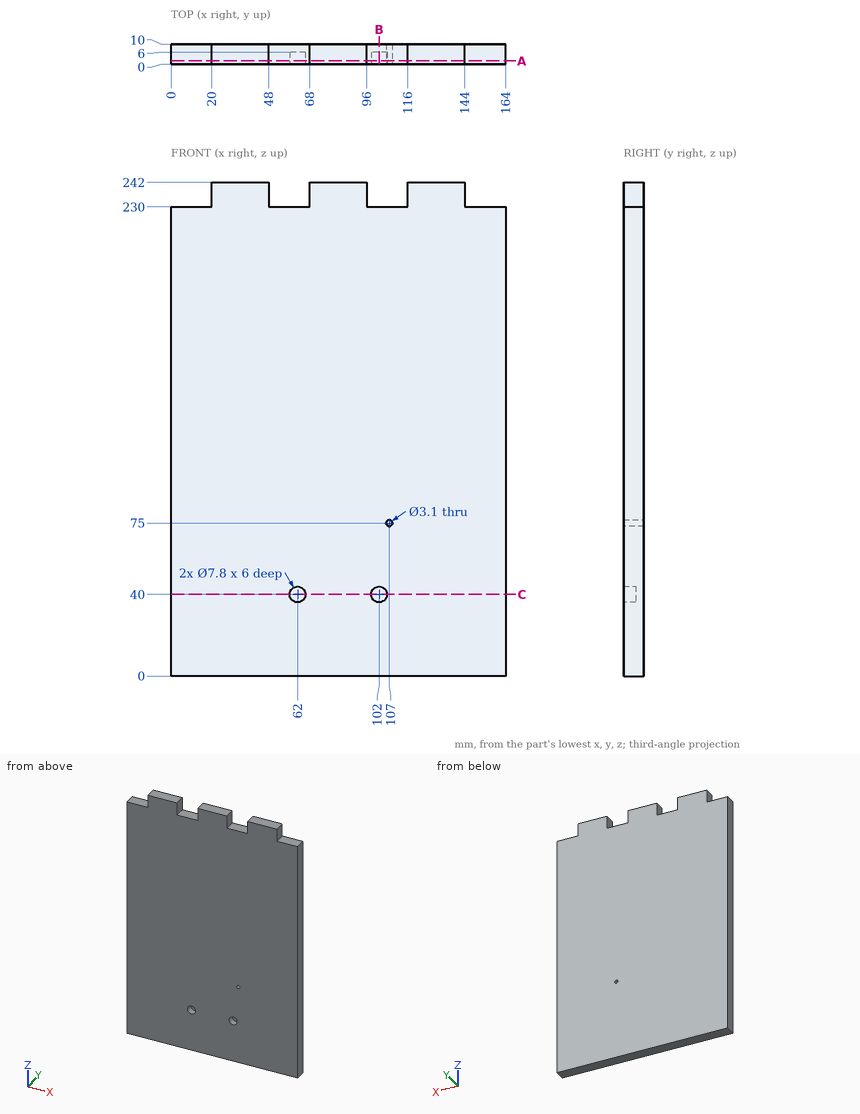
The drawing under review shows one solid part. Ordinate dimensions are in mm from its lowest x, y, z. Coordinates: 2 decimals unless noted, no trailing zeros. Order: outer loops, then holes, each group sorted by start corner. A loop starts at its lowest first (then second) coordinate and runs counter-clockwise, first axis right, second up. Notation, with made-up numbers: (42, -17) - (82, -17) arc R21 cw to (82, -3) - close; hole circle Ø3 at (57, 86.25). An arc over 180 degrees is marked (long way). Put each result on its own line as item: value.
1) Take a section at B-B, the plane x = 102. Give the boundary of the cut face in (y, z), and give its area (3 significant figures).
Response values:
outline: (0, 0) - (10, 0) - (10, 230) - (0, 230) - (0, 43.9) - (6, 43.9) - (6, 36.1) - (0, 36.1) - close
area: 2,250 mm²
2) Insertion check: P1, Ø3, axis at y = 6.5, z = 235.5, coming from the -X side; P2, Ø5, axis at x = 156, y = 5.5, coming from the +Z side; P3, Ø6, axis at x = 102, z = 40, coming from the -Y side. Each pin has a flat end and moves straight along its axis. Give the tip position at first contact, or say it passes through.
Response values:
P1: stops at x = 20
P2: stops at z = 230
P3: stops at y = 6
3) Wall thickness on L1, parallel to X at y = 4.25, z = 40; L2, parallel to X at y = 2.25, z = 75; L3, parallel to Z at x = 107, y = 7.25: over which ranges is each line inside the solid? List them lowest first. Write a range as from..to.
Response values:
L1: x = 0..58.1, 65.9..98.1, 105.9..164
L2: x = 0..105.45, 108.55..164
L3: z = 0..73.45, 76.55..230
4) Take a section at C-C, the plane z = 40. Give the boundary of the cut face in (x, y).
Response values:
outline: (0, 0) - (58.1, 0) - (58.1, 6) - (65.9, 6) - (65.9, 0) - (98.1, 0) - (98.1, 6) - (105.9, 6) - (105.9, 0) - (164, 0) - (164, 10) - (0, 10) - close
5) Take a section at A-A, the plane y = 1.75. Give the boundary of the cut face in (x, z), and give its area (3 significant figures).
Response values:
outline: (0, 0) - (164, 0) - (164, 230) - (144, 230) - (144, 242) - (116, 242) - (116, 230) - (96, 230) - (96, 242) - (68, 242) - (68, 230) - (48, 230) - (48, 242) - (20, 242) - (20, 230) - (0, 230) - close; hole circle Ø7.8 at (62, 40); hole circle Ø7.8 at (102, 40); hole circle Ø3.1 at (107, 75)
area: 38,600 mm²
